```python
from build123d import *

# Parameters (mm, degrees)
EXTRUDE_1_DEPTH     = 3
SKETCH_3_R          = 4
CUT_EXTRUDE_1_DEPTH = 2.5
FILLET_START        = -1
FILLET_1_DEPTH      = 5
FILLET_1_2_DEPTH    = 3
FILLET_2_R          = 6
SKETCH_4_R          = 4
CUT_EXTRUDE_2_DEPTH = 4
SKETCH_5_R          = 1.5
CUT_EXTRUDE_4_DEPTH = 10
SKETCH_6_R          = 2
CUT_EXTRUDE_5_DEPTH = 10


with BuildPart() as part:
    # 草图1 → 凸台-拉伸1 (new body)
    with BuildSketch(Plane.XY):
        with BuildLine():
            Line((0, 0), (80.101020514, 0))
            ThreePointArc((80.101020514, 0), (85, -2), (89.898979486, 0))
            Line((89.898979486, 0), (110.101020514, 0))
            ThreePointArc((110.101020514, 0), (122, 5), (110.101020514, 10))
            Line((110.101020514, 10), (89.898979486, 10))
            ThreePointArc((89.898979486, 10), (85, 12), (80.101020514, 10))
            Line((80.101020514, 10), (6, 10))
            Line((6, 10), (6, 28))
            Line((6, 28), (16, 28))
            Line((16, 28), (16, 34))
            Line((16, 34), (0, 34))
            Line((0, 34), (0, 0))
        make_face()
    extrude(amount=EXTRUDE_1_DEPTH)

    # 草图3 → 切除-拉伸1 (cut)
    with BuildSketch(Plane.XY.offset(3)):
        with Locations((115, 5)):
            Circle(SKETCH_3_R)
    extrude(amount=-CUT_EXTRUDE_1_DEPTH, mode=Mode.SUBTRACT)

    # 圆角1: read off the stored shape, not the designer's step
    # 圆角1 outline → 圆角1 (cut)
    with BuildSketch(Plane.XY.offset(FILLET_START)):
        with BuildLine():
            ThreePointArc((13, 34), (15.121320344, 33.121320344), (16, 31))
            Line((16, 31), (16, 34))
            Line((16, 34), (13, 34))
        make_face()
        with BuildLine():
            ThreePointArc((16, 31), (15.121320344, 28.878679656), (13, 28))
            Line((13, 28), (16, 28))
            Line((16, 28), (16, 31))
        make_face()
    extrude(amount=FILLET_1_DEPTH, mode=Mode.SUBTRACT)

    # Fillet 1 2 outline → Fillet 1 2 (add)
    with BuildSketch(Plane.XY):
        with BuildLine():
            Line((6, 28), (6, 25))
            ThreePointArc((6, 25), (6.878679656, 27.121320344), (9, 28))
            Line((9, 28), (6, 28))
        make_face()
        with BuildLine():
            ThreePointArc((9, 10), (6.878679656, 10.878679656), (6, 13))
            Line((6, 13), (6, 10))
            Line((6, 10), (9, 10))
        make_face()
    extrude(amount=FILLET_1_2_DEPTH)

    # 圆角2
    fillet_2_edges = [part.edges().sort_by_distance(p)[0] for p in [
        (0, 34, 1.5),
        (0, 0, 1.5),
    ]]
    fillet(fillet_2_edges, radius=FILLET_2_R)

    # 草图4 → 切除-拉伸2 (cut)
    with BuildSketch(Plane.XY.offset(3)):
        with Locations((85, 5)):
            Circle(SKETCH_4_R)
    extrude(amount=-CUT_EXTRUDE_2_DEPTH, mode=Mode.SUBTRACT)

    # 草图5 → 切除-拉伸4 (cut)
    with BuildSketch(Plane.XY):
        with Locations((75, 5)):
            Circle(SKETCH_5_R)
        with Locations((3, 10)):
            Circle(SKETCH_5_R)
        with Locations((13, 31)):
            Circle(SKETCH_5_R)
        with Locations((6, 31)):
            Circle(SKETCH_5_R)
    extrude(amount=CUT_EXTRUDE_4_DEPTH, mode=Mode.SUBTRACT)

    # 草图6 → 切除-拉伸5 (cut)
    with BuildSketch(Plane(origin=(0, 0, 0), x_dir=(-1, 0, 0), z_dir=(0, 0, -1))):
        with Locations((-115, 5)):
            Circle(SKETCH_6_R)
    extrude(amount=-CUT_EXTRUDE_5_DEPTH, mode=Mode.SUBTRACT)


solid = part.part
```
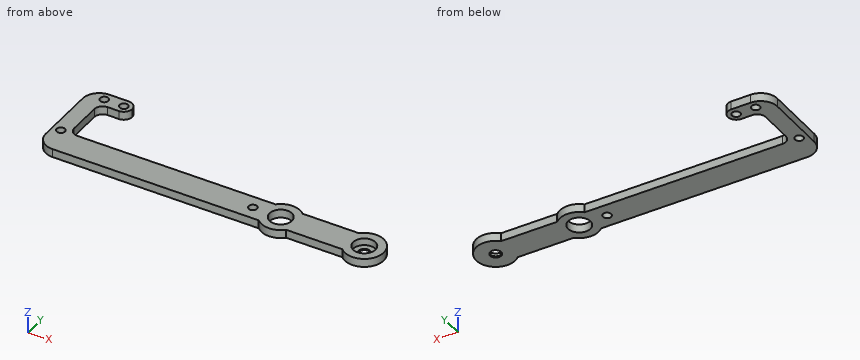
Geometry: final body of the model. Coordinates: model frame, mm. Give positions to 0.01 mm unless a question says otherwise; leave off trailing zeros. Loops run counter-clockwise (first coordinate to the right, second up) from the corner with the lowest first, then second, coordinate; pieces in that order, holes last. Notation, with made-up numbers: (41, 18.25) -> (53, 18.25) arc R19 ccw to (53, 32.25) -> close; hole circle Ø2 at (-24.5, -30.75). An arc over 180 degrees is marked (long way). Return JSON: item names as keys, results as strings.
Item 1: Section C-C, the plane x = 85. Output: boundary loops of the cut face in (y, z).
Filled in:
{"outline": "(-2, 0) -> (1, 0) -> (1, 3) -> (-2, 3) -> close; (9, 0) -> (12, 0) -> (12, 3) -> (9, 3) -> close"}
Item 2: Section A-A, the plane x = 115. Output: boundary loops of the cut face in (y, z).
Filled in:
{"outline": "(-2, 0) -> (3, 0) -> (3, 0.5) -> (1, 0.5) -> (1, 3) -> (-2, 3) -> close; (7, 0) -> (12, 0) -> (12, 3) -> (9, 3) -> (9, 0.5) -> (7, 0.5) -> close"}
Item 3: Section B-B, the plane z = 1.6. Output: boundary loops of the cut face in (x, y).
Filled in:
{"outline": "(0, 6) arc R6 ccw to (6, 0) -> (80.1, 0) arc R7 ccw to (89.9, 0) -> (110.1, 0) arc R7 ccw (long way) to (110.1, 10) -> (89.9, 10) arc R7 ccw to (80.1, 10) -> (9, 10) arc R3 cw to (6, 13) -> (6, 25) arc R3 cw to (9, 28) -> (13, 28) arc R3 ccw to (13, 34) -> (6, 34) arc R6 ccw to (0, 28) -> close; hole circle Ø3 at (3, 10); hole circle Ø3 at (6, 31); hole circle Ø3 at (13, 31); hole circle Ø3 at (75, 5); hole circle Ø8 at (85, 5); hole circle Ø8 at (115, 5)"}
Item 4: Section D-D, the plane x = 64.5. Output: boundary loops of the cut face in (y, z), plus the area to 3 significant figures.
Filled in:
{"outline": "(0, 0) -> (10, 0) -> (10, 3) -> (0, 3) -> close", "area": "30.0 mm^2"}
Item 5: Pin query (flat end, axial travel): P1, Ø5, axis at x = 75, y = 5, coming from the -Z side; P2, Ø1.8, axis at x = 13, y = 31, coming from the +Z side; P3, Ø1.5, axis at x = 12, z = 2, coming from the -Y side; P4, Ø1.5, axis at y = 18.5, z = 1.5, coming from the +X side. Return the tip coordinate at first contact, or that it passes through.
Filled in:
{"P1": "z = 0", "P2": "through", "P3": "y = 0", "P4": "x = 6"}
Item 6: Line query: line 1 (Y direction, x = 115, z = 2.3); line 2 (X direction, y = 32, z = 1.55); line 3 (Y direction, x = 115, z = 0.3). Output: solid intervals per line, ascending.
Filled in:
{"line 1": "-2 to 1, 9 to 12", "line 2": "1.53 to 4.88, 7.12 to 11.88, 14.12 to 15.83", "line 3": "-2 to 3, 7 to 12"}
